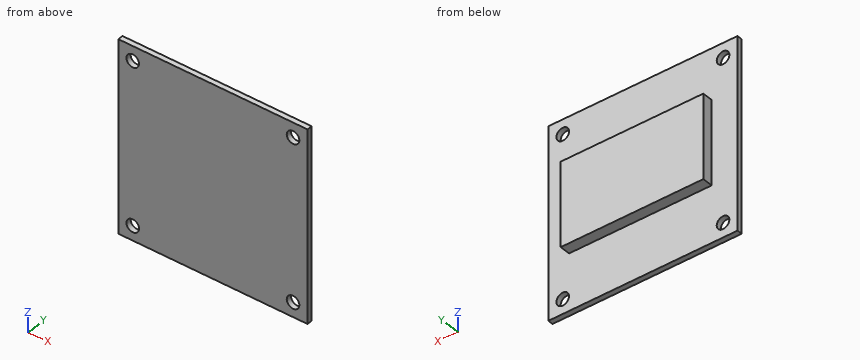
from build123d import *

# Parameters (mm, degrees)
ESQUISSE1_W        = 36
ESQUISSE1_H        = 36
BOSS_EXTRU_1_DEPTH = 1
D_GAGEMENT_M21_D   = 2.4
ESQUISSE4_W        = 27.125417606
ESQUISSE4_H        = 15.817725109
BOSS_EXTRU_2_DEPTH = 2


with BuildPart() as part:
    # Esquisse1 → Boss.-Extru.1 (new body)
    with BuildSketch(Plane(origin=(0, 0, 0), x_dir=(1, 0, 0), z_dir=(0, 1, 0))):
        with Locations((18, 18)):
            Rectangle(ESQUISSE1_W, ESQUISSE1_H)
    extrude(amount=BOSS_EXTRU_1_DEPTH)

    # Dégagement M21 (through all)
    with Locations(Plane(origin=(0, 1, 0), x_dir=(1, 0, 0), z_dir=(0, 1, 0))):
        with Locations((2.75, 2.75), (2.75, 33.25), (33.25, 33.25), (33.25, 2.75)):
            Hole(D_GAGEMENT_M21_D / 2)

    # Esquisse4 → Boss.-Extru.2 (add)
    with BuildSketch(Plane(origin=(0, 1, 0), x_dir=(1, 0, 0), z_dir=(0, 1, 0))):
        with Locations((18.47521777, 17.448351925)):
            Rectangle(ESQUISSE4_W, ESQUISSE4_H)
    extrude(amount=BOSS_EXTRU_2_DEPTH)


solid = part.part
Work out the finished part from the listing and answer in its coordinate system (mm). Coordinates: 2 decimals unless noted, no trailing zeros. Write each loop counter-clockwise with the first axis right and the second up, starting at its lowest first coordinate (ties: lowest second). Pieces come first, ordered by that corner, then holes. Notation, with made-up numbers: M 19,39.25 L 46,39.25 A13 ccw 46,49.25 Z; hole C 25.25,33 d3. An arc over 180 degrees is marked long. Answer as CSV lines item,"result". Start each with the question number.
Item 1: Section A-A on z = -2.75 is taken. Write down the section's boundary in (x, y), and give its area (3 significant figures).
Item 2: Section C-C on z = -13 is taken. Write down the section's boundary in (x, y).
Item 3: Section B-B on x = 2.75 is taken. Write down the section's boundary in (y, z).
Item 4: Consider L1, parallel to Z at x = 2.75, y = 0.6; L2, parallel to X at y = 0.2, z = -33.25; L3, parallel to Y at x = 33.5, z = -6.5. Determine where each line is inside the solid, lowest interval first.
Item 5: Flat-ended cylindrical pins translate along their axes: P1, Ø2, axis at x = 28.5, z = -8.5, coming from the +Y side; P2, Ø1, axis at y = 2, z = -18, coming from the -X side; P3, Ø1.6, axis at x = 21, y = 2.5, coming from the -Z side. Find the tip coordinate at first contact, or state that the pin passes through.
Item 6: Section D-D on y = 2.1 is taken. Write down the section's boundary in (x, z).
Checks:
1,outline,"M 0,0 L 1.55,0 L 1.55,1 L 0,1 Z; M 3.95,0 L 32.05,0 L 32.05,1 L 3.95,1 Z; M 34.45,0 L 36,0 L 36,1 L 34.45,1 Z"
1,area,"31.2 mm²"
2,outline,"M 0,0 L 36,0 L 36,1 L 32.04,1 L 32.04,3 L 4.91,3 L 4.91,1 L 0,1 Z"
3,outline,"M 0,-36 L 1,-36 L 1,-34.45 L 0,-34.45 Z; M 0,-32.05 L 1,-32.05 L 1,-3.95 L 0,-3.95 Z; M 0,-1.55 L 1,-1.55 L 1,0 L 0,0 Z"
4,L1,"z = -36 to -34.45, -32.05 to -3.95, -1.55 to 0"
4,L2,"x = 0 to 1.55, 3.95 to 32.05, 34.45 to 36"
4,L3,"y = 0 to 1"
5,P1,"stops at y = 1"
5,P2,"stops at x = 4.91"
5,P3,"stops at z = -25.36"
6,outline,"M 4.91,-25.36 L 32.04,-25.36 L 32.04,-9.54 L 4.91,-9.54 Z"
